CAD build for the part. Positions are in the model's coordinates, mm. A direction names the side the tool comes from. Round coordinates to 2 decimals unless told otherwise and drop trailing zeros. Loops run counter-clockwise (first coordinate to the right, second up) from the corner with the lowest first, then second, coordinate; pieces in that order, holes last. Notation, with made-up numbers: M 24.25,-30.75 L 57.25,-30.75 A25 cw 57.25,-0.75 Z; hole C -14.5,82.5 d7. An arc over 180 degrees is marked long. One line per item, written item: value. Start each with the question number.
from build123d import *

# Parameters (mm, degrees)
F0_R            = 23.8125
F0_R_2          = 2.15265
F0_R_3          = 14.2875
F1_DEPTH        = 7.9375
F3_DEPTH        = 7.9375
F3_COPIES_COUNT = 4
F4_R            = 23.8125
F4_R_2          = 2.15265
F4_R_3          = 14.2875
F4_R_4          = 12.7
F5_DEPTH        = 2.8575


# Not quite as in the source:
# - a pattern or mirror of a feature is missing from the dataset's text; its kind, count and spacing are read off the source's solid


with BuildPart() as f1:
    # F0 (on Top) → F1 (new body)
    with BuildSketch(Plane.XY):
        Circle(F0_R)
        with Locations((-13.4703841816, -13.4703841816)):
            Circle(F0_R_2, mode=Mode.SUBTRACT)
        with Locations((13.4703841816, -13.4703841816)):
            Circle(F0_R_2, mode=Mode.SUBTRACT)
        with Locations((-13.4703841816, 13.4703841816)):
            Circle(F0_R_2, mode=Mode.SUBTRACT)
        Circle(F0_R_3, mode=Mode.SUBTRACT)
        with Locations((13.4703841816, 13.4703841816)):
            Circle(F0_R_2, mode=Mode.SUBTRACT)
    extrude(amount=F1_DEPTH)

    # F2 (on face) → F3 (cut, through all)
    with BuildSketch(Plane.XY.offset(7.9375)):
        with BuildLine():
            ThreePointArc((12.7805200237, -18.1826547271), (10.4181406182, -17.1262309344), (8.9569606825, -14.9903889737))
            ThreePointArc((8.9569606825, -14.9903889737), (0, -17.4625), (-8.9569606825, -14.9903889737))
            ThreePointArc((-8.9569606825, -14.9903889737), (-10.4181406182, -17.1262309344), (-12.7805200237, -18.1826547271))
            ThreePointArc((-12.7805200237, -18.1826547271), (0, -22.225), (12.7805200237, -18.1826547271))
        make_face()
    f3 = extrude(amount=-F3_DEPTH, mode=Mode.SUBTRACT)

    # F3_copies: F3 ×4 about axis
    f3_copies_axis = Axis((0, 0, 0), (0, 0, 1))
    for i in range(1, F3_COPIES_COUNT):
        add(f3.rotate(f3_copies_axis, i * 360 / F3_COPIES_COUNT), mode=Mode.SUBTRACT)

    # F4 (on face) → F5 (join)
    with BuildSketch(Plane.XY.offset(7.9375)):
        Circle(F4_R)
        with Locations((-13.4703841816, -13.4703841816)):
            Circle(F4_R_2, mode=Mode.SUBTRACT)
        with BuildLine():
            ThreePointArc((-8.9569606825, -14.9903889737), (0, -17.4625), (8.9569606825, -14.9903889737))
            ThreePointArc((8.9569606825, -14.9903889737), (10.4181406182, -17.1262309344), (12.7805200237, -18.1826547271))
            ThreePointArc((12.7805200237, -18.1826547271), (0, -22.225), (-12.7805200237, -18.1826547271))
            ThreePointArc((-12.7805200237, -18.1826547271), (-10.4181406182, -17.1262309344), (-8.9569606825, -14.9903889737))
        make_face(mode=Mode.SUBTRACT)
        with Locations((13.4703841816, -13.4703841816)):
            Circle(F4_R_2, mode=Mode.SUBTRACT)
        with BuildLine():
            ThreePointArc((-14.9903889737, 8.9569606825), (-17.4625, 0), (-14.9903889737, -8.9569606825))
            ThreePointArc((-14.9903889737, -8.9569606825), (-17.1262309344, -10.4181406182), (-18.1826547271, -12.7805200237))
            ThreePointArc((-18.1826547271, -12.7805200237), (-22.225, 0), (-18.1826547271, 12.7805200237))
            ThreePointArc((-18.1826547271, 12.7805200237), (-17.1262309344, 10.4181406182), (-14.9903889737, 8.9569606825))
        make_face(mode=Mode.SUBTRACT)
        with Locations((-13.4703841816, 13.4703841816)):
            Circle(F4_R_2, mode=Mode.SUBTRACT)
        Circle(F4_R_3, mode=Mode.SUBTRACT)
        with BuildLine():
            ThreePointArc((14.9903889737, -8.9569606825), (17.4625, 0), (14.9903889737, 8.9569606825))
            ThreePointArc((14.9903889737, 8.9569606825), (17.1262309344, 10.4181406182), (18.1826547271, 12.7805200237))
            ThreePointArc((18.1826547271, 12.7805200237), (22.225, 0), (18.1826547271, -12.7805200237))
            ThreePointArc((18.1826547271, -12.7805200237), (17.1262309344, -10.4181406182), (14.9903889737, -8.9569606825))
        make_face(mode=Mode.SUBTRACT)
        with BuildLine():
            ThreePointArc((8.9569606825, 14.9903889737), (0, 17.4625), (-8.9569606825, 14.9903889737))
            ThreePointArc((-8.9569606825, 14.9903889737), (-10.4181406182, 17.1262309344), (-12.7805200237, 18.1826547271))
            ThreePointArc((-12.7805200237, 18.1826547271), (0, 22.225), (12.7805200237, 18.1826547271))
            ThreePointArc((12.7805200237, 18.1826547271), (10.4181406182, 17.1262309344), (8.9569606825, 14.9903889737))
        make_face(mode=Mode.SUBTRACT)
        with Locations((13.4703841816, 13.4703841816)):
            Circle(F4_R_2, mode=Mode.SUBTRACT)
        with BuildLine():
            ThreePointArc((12.7805200237, -18.1826547271), (10.4181406182, -17.1262309344), (8.9569606825, -14.9903889737))
            ThreePointArc((8.9569606825, -14.9903889737), (0, -17.4625), (-8.9569606825, -14.9903889737))
            ThreePointArc((-8.9569606825, -14.9903889737), (-10.4181406182, -17.1262309344), (-12.7805200237, -18.1826547271))
            ThreePointArc((-12.7805200237, -18.1826547271), (0, -22.225), (12.7805200237, -18.1826547271))
        make_face()
        with BuildLine():
            ThreePointArc((-18.1826547271, -12.7805200237), (-17.1262309344, -10.4181406182), (-14.9903889737, -8.9569606825))
            ThreePointArc((-14.9903889737, -8.9569606825), (-17.4625, 0), (-14.9903889737, 8.9569606825))
            ThreePointArc((-14.9903889737, 8.9569606825), (-17.1262309344, 10.4181406182), (-18.1826547271, 12.7805200237))
            ThreePointArc((-18.1826547271, 12.7805200237), (-22.225, 0), (-18.1826547271, -12.7805200237))
        make_face()
        Circle(F4_R_3)
        Circle(F4_R_4, mode=Mode.SUBTRACT)
        with BuildLine():
            ThreePointArc((18.1826547271, 12.7805200237), (17.1262309344, 10.4181406182), (14.9903889737, 8.9569606825))
            ThreePointArc((14.9903889737, 8.9569606825), (17.4625, 0), (14.9903889737, -8.9569606825))
            ThreePointArc((14.9903889737, -8.9569606825), (17.1262309344, -10.4181406182), (18.1826547271, -12.7805200237))
            ThreePointArc((18.1826547271, -12.7805200237), (22.225, 0), (18.1826547271, 12.7805200237))
        make_face()
        with BuildLine():
            ThreePointArc((-12.7805200237, 18.1826547271), (-10.4181406182, 17.1262309344), (-8.9569606825, 14.9903889737))
            ThreePointArc((-8.9569606825, 14.9903889737), (0, 17.4625), (8.9569606825, 14.9903889737))
            ThreePointArc((8.9569606825, 14.9903889737), (10.4181406182, 17.1262309344), (12.7805200237, 18.1826547271))
            ThreePointArc((12.7805200237, 18.1826547271), (0, 22.225), (-12.7805200237, 18.1826547271))
        make_face()
    extrude(amount=F5_DEPTH)


solid = f1.part
(1) Probe L1, parallel to Y at x = 0, z = 8.25; L2, parallel to Y at x = 0.5, z = 0.5; L3, parallel to Y at x = -10, z = 6. List the from-to ranges inside material, lowest first.
(2) Which spindle directions (+Z, -Z, +X, -X, +Y, -Y) get a long thin tool onto all of the face, cutting with end or side? Do faces 3 (the cylindrical face through (15.524, -12.824, 5.322)), 4 (the flat face through (-19, 0, 7.938)). Say none if no direction does.
(3) Slice it at C-C, the plane z = 6. Count the separate pieces of the cut face and the enclosed holes in it, and give its area (3 significant figures).
(4) Mould opens along Y. For faces 1 (the cylindrical face through (10.39, 17.1, 4.02)), 2 (the flat face through (10.25, -10.25, 0)) say: pulls with the +Y half, pulls with the -Y half, needs draft (parallel to the pull), parting line crosses it, or undercut.
(5) Slice it at A-A, the plane y = 0. List the corners of the cut face in (x, z) (1 decimal), and give its area (3 significant figures).
(6) Slice it at D-D, the plane z = 8.5. List the corners of the cut face in (x, y) (1 decimal).
(7) Flat gauge pins, fed straight in: P1, Ø3.5, axis at x = 19, y = 3.5, coming from the -Z side; P2, Ø23, axis at x = 0, y = 0, coming from the -Z side; P3, Ø1.5, axis at y = -9.5, z = 1, coming from the +X side; P4, Ø1, axis at x = -10, z = 2.5, coming from the -Y side. Where does each tip first touch, or does it go through?
Check result:
1. L1: y = -23.81 to -12.7, 12.7 to 23.81
1. L2: y = -23.81 to -22.22, -17.46 to -14.28, 14.28 to 17.46, 22.22 to 23.81
1. L3: y = -21.61 to -19.85, -16.73 to -10.2, 10.2 to 16.73, 19.85 to 21.61
2. face 3: +Z, -Z
2. face 4: -Z
3. separate pieces: 1
3. enclosed holes: 9
3. area: 662 mm^2
4. face 1: undercut
4. face 2: needs draft
5. outline: M -23.8,0 L -22.2,0 L -22.2,7.9 L -17.5,7.9 L -17.5,0 L -14.3,0 L -14.3,7.9 L -12.7,7.9 L -12.7,10.8 L -23.8,10.8 Z; M 12.7,7.9 L 14.3,7.9 L 14.3,0 L 17.5,0 L 17.5,7.9 L 22.2,7.9 L 22.2,0 L 23.8,0 L 23.8,10.8 L 12.7,10.8 Z
5. area: 139 mm^2
6. outline: C 0,0 d47.6; hole C -13.5,-13.5 d4.3; hole C -13.5,13.5 d4.3; hole C 0,0 d25.4; hole C 13.5,-13.5 d4.3; hole C 13.5,13.5 d4.3
7. P1: stops at z = 7.94
7. P2: passes through
7. P3: stops at x = 22.15
7. P4: stops at y = -21.84
